Part model, mm, in its own coordinate system. Face numbers are marked on the shaded views. A direction names the side the tool comes from. Round coordinates to 2 decimals unless told otherwise and drop trailing zeros. Loops run counter-clockwise (first coordinate to the right, second up) from the corner with the lowest first, then second, coordinate; pieces in that order, holes last.
1) Mould opens along X. For the marked faces 1, 2 and 3 say: +X half, -X half, draft (parallel to the pull), parting line (faces both ways), or undercut.
2) 3-axis set-ups, long thin cutter, end or side, ignore diameter. For the marked faces 4, 5 and 6: which of +Z, -Z, +X, -X, +Y, -Y reach the whole face in a straight line?
3) Drop flat-ended pins along their axis: P1, Ø1.5, axis at x = -7, z = 2.5, coming from the +Y side; P2, Ø1, axis at x = -3.5, z = 0.5, coming from the +Y side; P3, Ø1.5, axis at x = 5.5, z = 3, coming from the -Y side; P4, Ø4, axis at x = -7, y = -3, coming from the -Z side. Give the stop position or say it passes through.
4) Band-saw the part on C-C, the plane y = 8. Write the cut outline in (x, z), then the cut area to 3 significant figures.
5) Probe line 1 (Y direction, x = 0, z = 2.4); line 2 (Y direction, x = 15, z = 2.55); line 3 (Y direction, x = 14.5, z = 1.7). List the from-to ranges inside material, lowest first.
6) Band-saw the part on B-B, the plane x = -8.5. Write the cut outline in (y, z).
7) Band-saw the part on A-A, the plane y = 0. Write the cut outline in (x, z), then the cut area to 3 significant figures.
from build123d import *

# Parameters (mm, degrees)
F1_DEPTH = 4
F2_R     = 1.6
F3_DEPTH = 4.001


# Not quite as in the source:
# - ends of sketch curves that miss each other by under 0.0002 mm in the source are joined


with BuildPart() as f1:
    # F0 (on Top) → F1 (new body)
    with BuildSketch(Plane.XY):
        with BuildLine():
            ThreePointArc((1.9140106254, 14.2508572736), (1.6861265158, 14.1403198405), (1.4548574179, 14.2435879186))
            ThreePointArc((1.4548574179, 14.2435879186), (1.4306890387, 14.2754935862), (1.4109831428, 14.3103326425))
            Line((1.4109831428, 14.3103326425), (0.2558581901, 16.6921894723))
            ThreePointArc((0.2558581901, 16.6921894723), (0.1481039871, 16.8136670177), (-0.0071641706, 16.8612018631))
            ThreePointArc((-0.0071641706, 16.8612018631), (-0.1706127192, 16.817202235), (-0.2842271711, 16.6917305187))
            Line((-0.2842271711, 16.6917305187), (-1.4664410979, 14.2434227482))
            ThreePointArc((-1.4664410979, 14.2434227482), (-1.6902437576, 14.1388197245), (-1.916663057, 14.237631282))
            Line((-1.916663057, 14.237631282), (-3.6000092117, 16.3013673957))
            ThreePointArc((-3.6000092117, 16.3013673957), (-3.9019049125, 16.4036015506), (-4.125434594, 16.1763850942))
            Line((-4.125434594, 16.1763850942), (-4.7109828334, 13.5226488797))
            ThreePointArc((-4.7109828334, 13.5226488797), (-4.9015400565, 13.3688823231), (-5.1432019185, 13.4083253663))
            Line((-5.1432019185, 13.4083253663), (-7.2618513891, 15.0319710101))
            ThreePointArc((-7.2618513891, 15.0319710101), (-7.579185331, 15.0618374778), (-7.7442986009, 14.7892013747))
            Line((-7.7442986009, 14.7892013747), (-7.702174618, 12.0732144933))
            ThreePointArc((-7.702174618, 12.0732144933), (-7.8496947229, 11.8796668128), (-8.0921885063, 11.8591814286))
            Line((-8.0921885063, 11.8591814286), (-10.532310636, 12.9524153773))
            ThreePointArc((-10.532310636, 12.9524153773), (-10.8479798704, 12.9083044823), (-10.9457778263, 12.604942658))
            Line((-10.9457778263, 12.604942658), (-10.2788390418, 9.9731081586))
            ThreePointArc((-10.2788390418, 9.9731081586), (-10.375659889, 9.7510858631), (-10.6049250215, 9.6729470431))
            Line((-10.6049250215, 9.6729470431), (-13.2351231204, 10.1747796938))
            ThreePointArc((-13.2351231204, 10.1747796938), (-13.5321144192, 10.0590688256), (-13.5573261675, 9.7413311912))
            Line((-13.5573261675, 9.7413311912), (-12.3021100194, 7.3353788314))
            ThreePointArc((-12.3021100194, 7.3353788314), (-12.3432937572, 7.097610167), (-12.5462575743, 6.967089184))
            Line((-12.5462575743, 6.967089184), (-15.2246187544, 6.8487666996))
            ThreePointArc((-15.2246187544, 6.8487666996), (-15.4869255508, 6.6676921814), (-15.4381922857, 6.3527034427))
            Line((-15.4381922857, 6.3527034427), (-13.6629152877, 4.3020497532))
            ThreePointArc((-13.6629152877, 4.3020497532), (-13.6465657396, 4.062029571), (-13.8118007442, 3.8871742342))
            Line((-13.8118007442, 3.8871742342), (-16.3935721919, 3.153634337))
            ThreePointArc((-16.3935721919, 3.153634337), (-16.6070572662, 2.9169553146), (-16.4870055032, 2.621692024))
            Line((-16.4870055032, 2.621692024), (-14.2878546387, 1.0364711274))
            ThreePointArc((-14.2878546387, 1.0364711274), (-14.2152379851, 0.8077409694), (-14.3335516124, 0.5989526815))
            Line((-14.3335516124, 0.5989526815), (-16.6789818187, -0.7114654884))
            ThreePointArc((-16.6789818187, -0.7114654884), (-16.832139234, -0.9909930232), (-16.6472392521, -1.2506174313))
            Line((-16.6472392521, -1.2506174313), (-14.1431571391, -2.2854765977))
            ThreePointArc((-14.1431571391, -2.2854765977), (-14.0186393167, -2.4900607643), (-14.0835502146, -2.7205948066))
            Line((-14.0835502146, -2.7205948066), (-16.0654652706, -4.5382203487))
            ThreePointArc((-16.0654652706, -4.5382203487), (-16.1500404943, -4.8455310516), (-15.9102576154, -5.0555239268))
            Line((-15.9102576154, -5.0555239268), (-13.2365040498, -5.4848550701))
            ThreePointArc((-13.2365040498, -5.4848550701), (-13.0673141606, -5.6538228156), (-13.0753841374, -5.8928002059))
            Line((-13.0753841374, -5.8928002059), (-14.5860884781, -8.1203844463))
            ThreePointArc((-14.5860884781, -8.1203844463), (-14.5975232656, -8.4389155785), (-14.3157807663, -8.5879591986))
            Line((-14.3157807663, -8.5879591986), (-11.6166191171, -8.3893058066))
            ThreePointArc((-11.6166191171, -8.3893058066), (-11.4124537807, -8.5131996233), (-11.3634554587, -8.746935215))
            Line((-11.3634554587, -8.746935215), (-12.3205835531, -11.2648943843))
            ThreePointArc((-12.3205835531, -11.2648943843), (-12.258261618, -11.5774784738), (-11.9497442197, -11.6575400221))
            Line((-11.9497442197, -11.6575400221), (-9.3706481648, -10.8423342647))
            ThreePointArc((-9.3706481648, -10.8423342647), (-9.143139116, -10.914229028), (-9.0400495076, -11.1294074585))
            Line((-9.0400495076, -11.1294074585), (-9.3910515674, -13.8022744624))
            ThreePointArc((-9.3910515674, -13.8022744624), (-9.2583317968, -14.0920645572), (-8.9396672739, -14.0988290571))
            Line((-8.9396672739, -14.0988290571), (-6.6194690015, -12.711740107))
            ThreePointArc((-6.6194690015, -12.711740107), (-6.3815431901, -12.7276255469), (-6.2303634454, -12.912031956))
            Line((-6.2303634454, -12.912031956), (-5.955381825, -15.5957706951))
            ThreePointArc((-5.955381825, -15.5957706951), (-5.7594172495, -15.8471483428), (-5.4477802634, -15.7802512165))
            Line((-5.4477802634, -15.7802512165), (-3.5111841497, -13.8967395131))
            ThreePointArc((-3.5111841497, -13.8967395131), (-3.2763512695, -13.8557442651), (-3.0857625615, -13.9989330789))
            Line((-3.0857625615, -13.9989330789), (-2.1987423004, -16.54872127))
            ThreePointArc((-2.1987423004, -16.54872127), (-1.9500945765, -16.7481382853), (-1.6622810343, -16.6111850031))
            Line((-1.6622810343, -16.6111850031), (-0.2131467972, -14.3333958211))
            ThreePointArc((-0.2131467972, -14.3333958211), (0.005246929, -14.2378403367), (0.2243723928, -14.331705673))
            Line((0.2243723928, -14.331705673), (1.6764001268, -16.6097662074))
            ThreePointArc((1.6764001268, -16.6097662074), (1.9643299452, -16.746474862), (2.2128081189, -16.546846623))
            Line((2.2128081189, -16.546846623), (3.0970506062, -13.9980658779))
            ThreePointArc((3.0970506062, -13.9980658779), (3.286561705, -13.8533408388), (3.521767647, -13.8925576515))
            Line((3.521767647, -13.8925576515), (5.4611917751, -15.775615445))
            ThreePointArc((5.4611917751, -15.775615445), (5.7728854965, -15.8422477244), (5.9686363857, -15.5907036409))
            Line((5.9686363857, -15.5907036409), (6.2411397895, -12.9086763338))
            ThreePointArc((6.2411397895, -12.9086763338), (6.3909195318, -12.7229527682), (6.6288572495, -12.7052650163))
            Line((6.6288572495, -12.7052650163), (8.9516484854, -14.0912261582))
            ThreePointArc((8.9516484854, -14.0912261582), (9.2703071449, -14.0841908662), (9.4027806099, -13.7942880935))
            Line((9.4027806099, -13.7942880935), (9.0497770711, -11.1237609685))
            ThreePointArc((9.0497770711, -11.1237609685), (9.1511783498, -10.9075475026), (9.3783451778, -10.8338880535))
            Line((9.3783451778, -10.8338880535), (11.9596494988, -11.6473797597))
            ThreePointArc((11.9596494988, -11.6473797597), (12.268098751, -11.5670560686), (12.3301550361, -11.2544191321))
            Line((12.3301550361, -11.2544191321), (11.3716636637, -8.7393106928))
            ThreePointArc((11.3716636637, -8.7393106928), (11.4187295037, -8.5048818109), (11.6222137202, -8.3793180118))
            Line((11.6222137202, -8.3793180118), (14.3230763647, -8.5757891676))
            ThreePointArc((14.3230763647, -8.5757891676), (14.604692108, -8.4265061824), (14.5929866434, -8.1079848822))
            Line((14.5929866434, -8.1079848822), (13.0816946487, -5.8836056031))
            ThreePointArc((13.0816946487, -5.8836056031), (13.0715015116, -5.644332005), (13.2396929757, -5.4738404035))
            Line((13.2396929757, -5.4738404035), (15.9145504354, -5.0420000401))
            ThreePointArc((15.9145504354, -5.0420000401), (16.15415478, -4.8318034782), (16.0693184405, -4.5245647566))
            Line((16.0693184405, -4.5245647566), (14.0876977194, -2.7103070117))
            ThreePointArc((14.0876977194, -2.7103070117), (14.0205346934, -2.4799248131), (14.1437623045, -2.2740078751))
            Line((14.1437623045, -2.2740078751), (16.648298033, -1.2364685688))
            ThreePointArc((16.648298033, -1.2364685688), (16.8329773247, -0.9766871303), (16.6795824278, -0.6972898464))
            Line((16.6795824278, -0.6972898464), (14.335398798, 0.6098192161))
            ThreePointArc((14.335398798, 0.6098192161), (14.2147728105, 0.8179597828), (14.2858336525, 1.0477933771))
            Line((14.2858336525, 1.0477933771), (16.4847732853, 2.6357032988))
            ThreePointArc((16.4847732853, 2.6357032988), (16.6045740963, 2.9310685003), (16.3908879741, 3.1675660221))
            Line((16.3908879741, 3.1675660221), (13.8113473036, 3.8981036809))
            ThreePointArc((13.8113473036, 3.8981036809), (13.6438142546, 4.0717671277), (13.6583646175, 4.3126293336))
            Line((13.6583646175, 4.3126293336), (15.4327894801, 6.3658219818))
            ThreePointArc((15.4327894801, 6.3658219818), (15.4812550566, 6.6808520192), (15.2187944815, 6.8617035691))
            Line((15.2187944815, 6.8617035691), (12.5436443132, 6.9776065604))
            ThreePointArc((12.5436443132, 6.9776065604), (12.3384761371, 7.1063341886), (12.2952606451, 7.3446558284))
            Line((12.2952606451, 7.3446558284), (13.5490440665, 9.7528499611))
            ThreePointArc((13.5490440665, 9.7528499611), (13.5235623203, 10.0705660564), (13.2264728, 10.1860245057))
            Line((13.2264728, 10.1860245057), (10.6004372903, 9.6826728997))
            ThreePointArc((10.6004372903, 9.6826728997), (10.3691452759, 9.7583299946), (10.2700448298, 9.9805890632))
            Line((10.2700448298, 9.9805890632), (10.9350629039, 12.6142408462))
            ThreePointArc((10.9350629039, 12.6142408462), (10.8370071926, 12.9175194542), (10.5213005877, 12.961362084))
            Line((10.5213005877, 12.961362084), (8.0862749191, 11.8679259428))
            ThreePointArc((8.0862749191, 11.8679259428), (7.8420206158, 11.8850667554), (7.6918940409, 12.0784988717))
            Line((7.6918940409, 12.0784988717), (7.7317284499, 14.7957778483))
            ThreePointArc((7.7317284499, 14.7957778483), (7.566383559, 15.0682735431), (7.2490751116, 15.0381374223))
            Line((7.2490751116, 15.0381374223), (5.1365969535, 13.4163699229))
            ThreePointArc((5.1365969535, 13.4163699229), (4.8935343549, 13.3722272394), (4.6997550083, 13.5254511546))
            Line((4.6997550083, 13.5254511546), (4.1116867961, 16.1798854092))
            ThreePointArc((4.1116867961, 16.1798854092), (3.8879641114, 16.4069118327), (3.5861553961, 16.3044211699))
            Line((3.5861553961, 16.3044211699), (1.9140106254, 14.2508572736))
        make_face()
    extrude(amount=F1_DEPTH)

    # F2 (on face) → F3 (cut, through all)
    with BuildSketch(Plane.XY.offset(4)):
        Circle(F2_R)
    extrude(amount=-F3_DEPTH, mode=Mode.SUBTRACT)


solid = f1.part
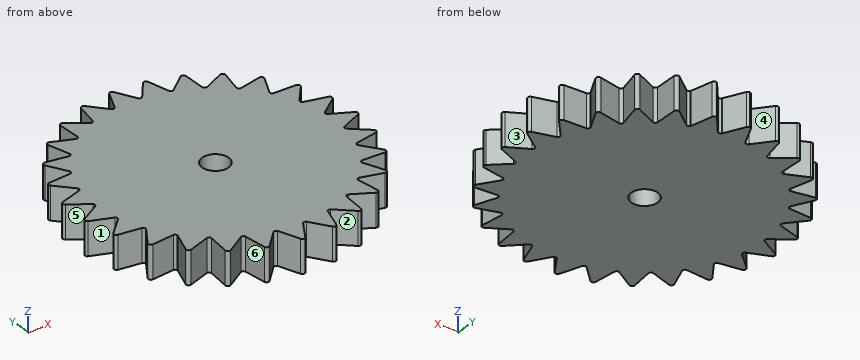
Reported:
1. face 1: -X half
1. face 2: undercut
1. face 3: +X half
2. face 4: +Z, -Z, +Y
2. face 5: +Z, -Z, -X
2. face 6: +Z, -Z, -Y
3. P1: stops at y = 15.09
3. P2: stops at y = 16.41
3. P3: stops at y = -15.86
3. P4: stops at z = 0
4. outline: (-12.65, 0) - (12.64, 0) - (12.64, 4) - (-12.65, 4) - close
4. area: 101 mm2
5. line 1: y = -14.24 to -1.6, 1.6 to 16.86
5. line 2: y = -5.19 to -3.55, -1.92 to 0.24, 1.56 to 3.56, 5.87 to 6.87
5. line 3: y = -8.53 to -7.97, -5.27 to -3.09, -2.13 to 0.52, 1.2 to 3.7, 5.29 to 6.89
6. outline: (-13.84, 0) - (12.04, 0) - (12.04, 4) - (-13.84, 4) - close
7. outline: (-15.41, 0) - (-1.6, 0) - (-1.6, 4) - (-15.41, 4) - close; (1.6, 0) - (15.43, 0) - (15.43, 4) - (1.6, 4) - close
7. area: 111 mm2
